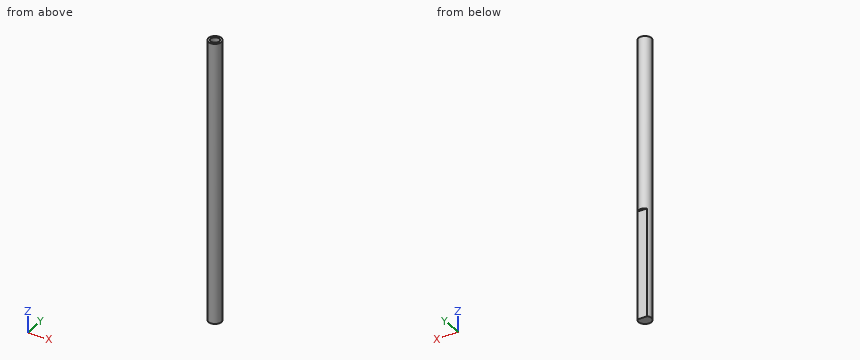
Autodesk Inventor part; units mm, degrees
ref_plane "YZ Plane" through (0, 0, 0) normal (1, 0, 0) x (0, 1, 0)
ref_plane "XZ Plane" through (0, 0, 0) normal (0, 1, 0) x (-1, 0, 0)
ref_plane "XY Plane" through (0, 0, 0) normal (0, 0, 1) x (1, 0, 0)
sketch "Sketch1" plane through (0, 0, 0) normal (0, 0, 1) x (1, 0, 0)
  circle A0 centre (0, 0) radius 3
  line L0 (-2.2361, 2) -> (2.2361, 2)
  arc A1 (-2.2361, 2) -> (2.2361, 2) centre (0, 0) ccw
  dimension "d0" = 6
  dimension "d1" = 2
extrude "Extrusion1" add sketch "Sketch1" along normal blind 130
sketch "Sketch3" plane through (0, 0, 130) normal (0, 0, 1) x (1, 0, 0)
  circle A0 centre (0, 0) radius 2
  dimension "d22" = 4
extrude "Extrusion3" cut sketch "Sketch3" against normal blind 12.7
sketch "Sketch4" plane through (0, 0, 0) normal (0, 0, -1) x (-1, 0, 0)
  circle A0 centre (0, 0) radius 3
  line L0 (-2.2361, 2) -> (2.2361, 2)
  arc A1 (-2.2361, 2) -> (2.2361, 2) centre (0, 0) ccw
  dimension "d25" = 2
extrude "Extrusion4" cut sketch "Sketch4" against normal blind 50 contours L0 A0 picked at (-0.5653, 2.1582)
properties part number "6mm x 160mm D Shaft" material "Stainless Steel"
Geometry check sheet. Reference: the model listing, model coordinates, mm. Coordinates: 2 decimals unless noted, no trailing zeros. Write each loop counter-clockwise with the first axis right and the second up, starting at its lowest first coordinate (ties: lowest second). Pieces come first, ordered by that corner, then holes. Notation, with made-up numbers: M 21,46.25 L 61,46.25 A28 ccw 61,71.25 Z; hole C 23,-8 d3. An arc over 180 degrees is marked long. Use one line per item in the form item = value. Start each with the question number.
1) Thickness scan on probe 1 along Y at (x, z) = (0, 123.25); probe 2 along Z at (x, y) = (-1.8, 0.65); probe 3 along Y at (x, z) = (-2, 88). Record the ranges inside material, lowest first. Write a range as from..to.
2) Section check A-A on x = 0. Enter the section's corners in (y, z), and give its area (3 significant figures).
3) Go/stop test with flat-tipped pins: pin 1 Ø3 at (x, y) = (0, 0) entering from +Z; pin 2 Ø1 at (x, z) = (1.5, 72.5) entering from -Y; pin 3 Ø0.5 at (x, y) = (0, 2.5) entering from -Z. Record where each tip stops, or that it passes through.
4) Section check B-B on y = 0. Enter the section's corners in (x, z), and give its area (3 significant figures).
5) Section check C-C on z = 88. Enter the section's corners in (x, y).
Responses:
q1.probe_1 = -3..-2, 2..3
q1.probe_2 = 0..117.3
q1.probe_3 = -2.24..2.24
q2.outline = M -3,0 L 2,0 L 2,50 L 3,50 L 3,130 L 2,130 L 2,117.3 L -2,117.3 L -2,130 L -3,130 Z
q2.area = 679 mm2
q3.pin_1 = 117.3
q3.pin_2 = -2.83
q3.pin_3 = 50
q4.outline = M -3,0 L 3,0 L 3,130 L 2,130 L 2,117.3 L -2,117.3 L -2,130 L -3,130 Z
q4.area = 729 mm2
q5.outline = C 0,0 d6
